Autodesk Inventor part; units mm, degrees
ref_plane "YZ Plane" through (0, 0, 0) normal (1, 0, 0) x (0, 1, 0)
ref_plane "XZ Plane" through (0, 0, 0) normal (0, 1, 0) x (-1, 0, 0)
ref_plane "XY Plane" through (0, 0, 0) normal (0, 0, 1) x (1, 0, 0)
sketch "Sketch1" plane through (0, 0, 0) normal (0, 1, 0) x (-1, 0, 0)
  circle A0 centre (0, 0) radius 10
  dimension "d0" = 20
extrude "Extrusion1" add sketch "Sketch1" along normal blind 15
sketch "Sketch2" plane through (0, 0, 0) normal (0, -1, 0) x (1, 0, 0)
  circle A0 centre (0, 0) radius 7.5
  dimension "d3" = 15
extrude "Extrusion2" cut sketch "Sketch2" against normal blind 5
fillet "Fillet1" radius 2 1 edges at (10, 15, 0)
sketch "Sketch4" plane through (0, 15, 0) normal (0, 1, 0) x (1, 0, 0)
  arc A0 (2.7981, -2.4967) -> (-1.483, -3.4443) centre (0, 0) ccw
  arc A1 (3.6613, -3.4051) -> (-2.1245, -4.5262) centre (0, 0) ccw
  line L0 (-2.1245, -4.5262) -> (-1.483, -3.4443)
  line L1 (1.8934, -3.9852) -> (2.2247, -1.8934)
  line L2 (4.2127, -3.9852) -> (1.8934, -3.9852)
  line L3 (2.2247, -1.8934) -> (2.7981, -2.4967)
  line L4 (3.6613, -3.4051) -> (4.2127, -3.9852)
  dimension "d12" = 7.5
  dimension "d13" = 10
extrude "Extrusion4" add sketch "Sketch4" along normal blind 0.5
properties part number "Device Rotation Button"
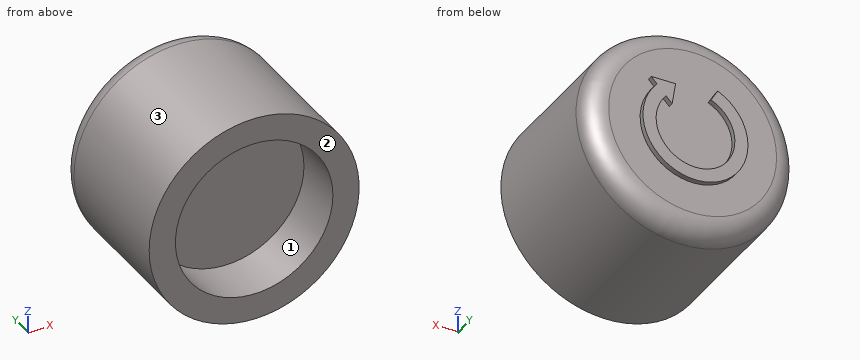
Read the model definition and answer for the solid it produces. Units are mm, in the model's axes. Face numbers are marked on the shaded views. Give positions to 0.01 mm unless a question says otherwise; leave off trailing zeros. Write each loop counter-clockwise with the first axis right and the second up, starting at its lowest first coordinate (ties: lowest second). Pieces come first, ordered by that corner, then holes. Notation, with made-up numbers: (15, 37.5) -> (42, 37.5) arc R25 cw to (42, 72.5) -> close; hole circle Ø10 at (8, 15). An arc over 180 degrees is marked (long way). Answer as a JSON object with one key per item and string values.
1) Section A-A on z = 0 is taken. Write down the section's boundary in (x, y), then the cut area to 3 significant figures.
Findings below:
{"outline": "(-10, 0) -> (-7.5, 0) -> (-7.5, 5) -> (7.5, 5) -> (7.5, 0) -> (10, 0) -> (10, 13) arc R2 ccw to (8, 15) -> (5, 15) -> (5, 15.5) -> (3.75, 15.5) -> (3.75, 15) -> (-3.75, 15) -> (-3.75, 15.5) -> (-5, 15.5) -> (-5, 15) -> (-8, 15) arc R2 ccw to (-10, 13) -> close", "area": "225 mm^2"}
2) Straight lines are drawn through the part: probe 1 along Z at (x, y) = (0, 2); probe 2 along Y at (x, z) = (-6.5, 1); probe 3 along Z at (x, y) = (-6.25, 4.5). For each, find the intervals that lie inside material, in ascending order. Write a range as from..to.
Findings below:
{"probe 1": "z = -10..-7.5, 7.5..10", "probe 2": "y = 5..15", "probe 3": "z = -7.81..-4.15, 4.15..7.81"}
3) For a pull along Z with two mould halves and no side action, classify the marked faces 1, 2 and 3 as pulls with the +Z half, pulls with the -Z half, needs draft (parallel to the pull), parting line crosses it, or undercut.
Findings below:
{"face 1": "undercut", "face 2": "needs draft", "face 3": "parting line crosses it"}
4) Section B-B on x = 0 is taken. Write down the section's boundary in (y, z).
Findings below:
{"outline": "(0, -10) -> (13, -10) arc R2 ccw to (15, -8) -> (15, -5) -> (15.5, -5) -> (15.5, -3.75) -> (15, -3.75) -> (15, 8) arc R2 ccw to (13, 10) -> (0, 10) -> (0, 7.5) -> (5, 7.5) -> (5, -7.5) -> (0, -7.5) -> close"}
5) Flat-ended cylindrical pins translate along their axes: pin 1 Ø4 at (x, y) = (5, 10.5) entering from -Z; pin 2 Ø8 at (y, z) = (5, -8) entering from +X; pin 3 Ø4 at (x, y) = (7, 3) entering from +Z. Find the tip coordinate at first contact, or state that the pin passes through.
Findings below:
{"pin 1": "stops at z = -9.54", "pin 2": "stops at x = 9.17", "pin 3": "stops at z = 8.66"}
6) Section C-C on y = 11.5 is taken. Write down the section's boundary in (x, z), then the cut area to 3 significant figures.
Findings below:
{"outline": "circle Ø20 at (0, 0)", "area": "314 mm^2"}
